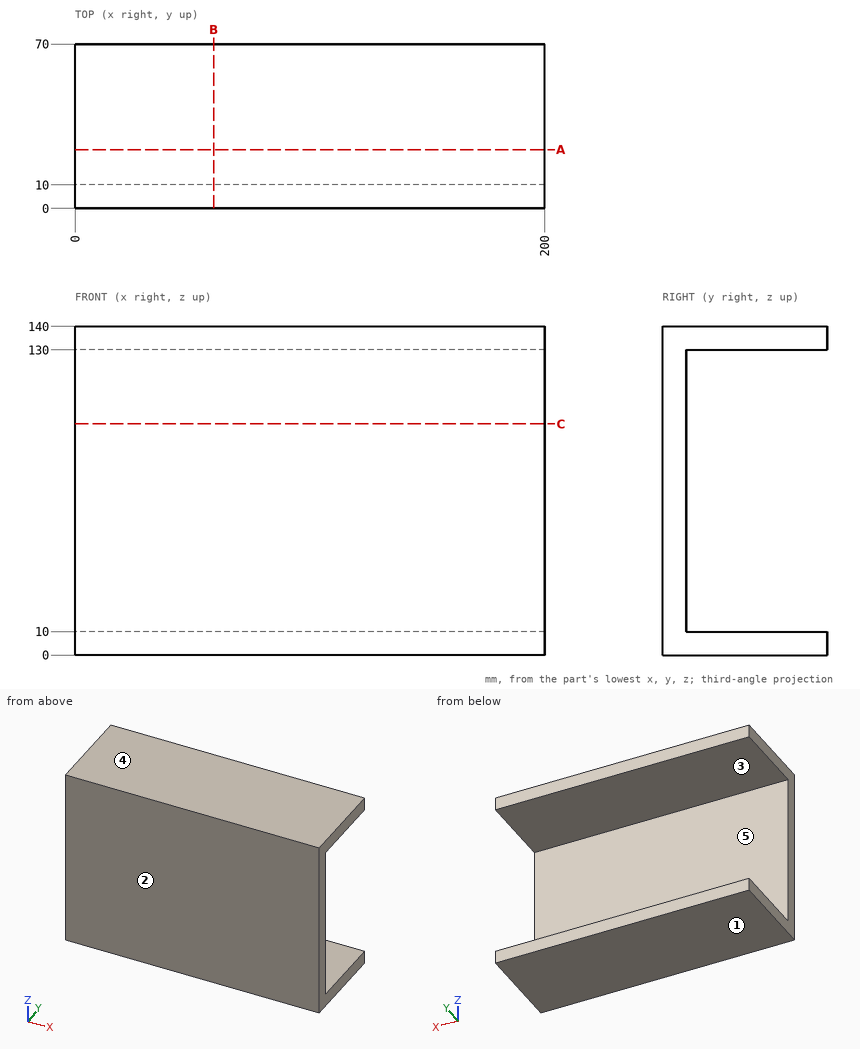
Answer from the drawing. Dimensions are ordinates in mm from the lowest x, y and z of the part. A direction names the side the tool comes from. Coordinates: 2 decimals unless noted, no trailing zeros. Loops run counter-clockwise (first coordinate to the right, second up) from the corner with the lowest first, then second, coordinate; pieces in that order, holes last. Notation, with made-up numbers: (64.5, 1.5) - (120.5, 1.5) arc R25 ccw to (120.5, 25.5) - close; hole circle Ø3 at (-23.5, 22). An arc over 180 degrees is marked (long way). Answer in a Markdown table with one row per item.
1. Determine the mould class of the marked faces 1, 2 and 3 for opening direction Z: +Z half, -Z half, draft (parallel to the pull), parting line (faces both ways), or undercut.
Conclusion:
| item | result |
|---|---|
| face 1 | -Z half |
| face 2 | draft |
| face 3 | undercut |
2. Find section B-B, the plane x = 59. Write down the section's boundary in (y, z), then the cut area to 3 significant figures.
Conclusion:
| item | result |
|---|---|
| outline | (0, 0) - (70, 0) - (70, 10) - (10, 10) - (10, 130) - (70, 130) - (70, 140) - (0, 140) - close |
| area | 2,600 mm² |
3. Find section C-C, the plane z = 98.5. Write down the section's boundary in (x, y).
Conclusion:
| item | result |
|---|---|
| outline | (0, 0) - (200, 0) - (200, 10) - (0, 10) - close |
4. Straight lines are drawn through the part: line 1 (Z direction, x = 68.5, y = 43); line 2 (Y direction, x = 66, z = 124). For each, find the intervals that lie inside material, in ascending order.
Conclusion:
| item | result |
|---|---|
| line 1 | z = 0 to 10, 130 to 140 |
| line 2 | y = 0 to 10 |
5. Given pin 1 (3 mm diameter, centred on x = 68.5, z = 99, fed in from +Y), flat-ended and moving along its own axis, determine where the tip first touches the part or whether it passes through.
Conclusion:
| item | result |
|---|---|
| pin 1 | stops at y = 10 |
6. Which of the six approach directions +Z, -Z, +X, -X, +Y, -Y give full straight-line access (tool end or side, diameter ignored) to the marked faces 4 and 5?
Conclusion:
| item | result |
|---|---|
| face 4 | +Z, +X, -X, +Y, -Y |
| face 5 | +X, -X, +Y |
7. Find section A-A, the plane y = 25. Write down the section's boundary in (x, z).
Conclusion:
| item | result |
|---|---|
| outline | (0, 0) - (200, 0) - (200, 10) - (0, 10) - close; (0, 130) - (200, 130) - (200, 140) - (0, 140) - close |
